The model under review builds one solid part; all positions refer to its coordinate system, in mm. Face numbers are marked on the shaded views. Coordinates: 2 decimals unless noted, no trailing zeros. Write each loop counter-clockwise with the first axis right and the second up, starting at its lowest first coordinate (ties: lowest second). Pieces come first, ordered by that corner, then holes.
1) For line 1 (Y direction, x = 0, z = 0.05); line 2 (Y direction, x = 28.5, z = 3.75); line 3 (Z direction, x = 6.5, y = -12), list the stretches that pass through material, from the lowest coordinate up.
2) Add section A-A, the plane z = 13. State the section outline as (x, y) points, then the cut area to 3 significant figures.
3) Mouldability with a two-part tool opening along X and no side actions: class the marked faces 1, 2 and 3 as released by +X, released by -X, zero draft, split by the parting line, or undercut.
4) For P1, Ø1, axis at y = 21.5, z = 2, coming from the -X side; P2, Ø5, axis at y = -2.5, z = 10.5, coming from the +X side; P3, Ø4, axis at y = 15.5, z = 4, coming from the -X side; P4, Ø4, axis at y = 20.5, z = 12.5, coming from the +X side, all flat-tipped, find the tip position at first contact; note any pin that passes through.
5) Add section B-B, the plane z = 3.25. State the section outline as (x, y) points, then the cut area to 3 significant figures.
from build123d import *

# Parameters (mm, degrees)
F0_R     = 40
F1_DEPTH = 15
F2_SIZE  = 5
F3_R     = 25
F4_DEPTH = 10
F5_SIZE2 = 9.99999
F5_SIZE  = 24.99999


# Not quite as in the source:
# - a fillet or chamfer is up to 0.001 mm smaller than in the source, because OpenCascade refuses the exact size


with BuildPart() as f1:
    # F0 (on Top) → F1 (new body)
    with BuildSketch(Plane.XY):
        Circle(F0_R)
    extrude(amount=F1_DEPTH)

    # F2
    f2_edges = [f1.edges().sort_by_distance(p)[0] for p in [
        (-40, 0, 15),
    ]]
    chamfer(f2_edges, length=F2_SIZE)

    # F3 (on face) → F4 (cut)
    with BuildSketch(Plane(origin=(0, 0, 0), x_dir=(1, 0, 0), z_dir=(0, 0, -1))):
        Circle(F3_R)
    extrude(amount=-F4_DEPTH, mode=Mode.SUBTRACT)

    # F5 (size 25 and 10 in the source; OpenCascade refuses exactly that, so slightly less here)
    f5_edges = [f1.edges().sort_by_distance(p)[0] for p in [
        (-25, 0, 10),
    ]]
    f5_side = f1.faces().sort_by_distance((0, 0, 10))[0]
    chamfer(f5_edges, length=F5_SIZE, length2=F5_SIZE2, reference=f5_side)


solid = f1.part
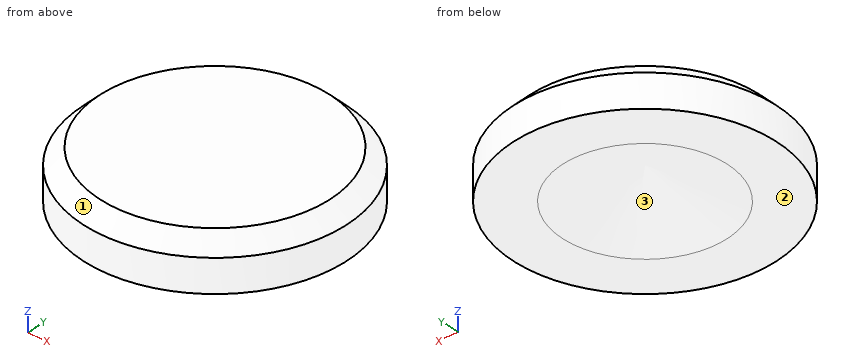
Geometry results:
1. line 1: y = -40 to -24.88, 24.88 to 40
1. line 2: y = -28.07 to 28.07
1. line 3: z = 4.54 to 15
2. outline: circle Ø74 at (0, 0)
2. area: 4,300 mm2
3. face 1: split by the parting line
3. face 2: zero draft
3. face 3: undercut
4. P1: stops at x = -34.04
4. P2: stops at x = 40
4. P3: stops at x = -37.65
4. P4: stops at x = 34.05
5. outline: circle Ø80 at (0, 0); hole circle Ø33.75 at (0, 0)
5. area: 4,130 mm2
